Can you work these out from the model? Positions are in its coordinate system, mm. Face numbers are marked on the shaded views. A direction names the side the tool comes from. Coordinates: 2 decimals unless noted, no trailing zeros. Loops run counter-clockwise (first coordinate to the right, second up) from the corner with the lowest first, then second, coordinate; pieces in that order, holes last. Notation, with made-up numbers: (-30, 0.25) -> (-8, 0.25) arc R26 ccw to (-8, 31.25) -> close; hole circle Ø10 at (-36, 30.25). An arc over 180 degrees is marked (long way). Use one line per item in the form item = value. Start each with the question number.
(1) Imagine slicing it at B-B (y = -31). State how many separate pieces and enclosed holes the cut face has, plus the area to 3 significant figures.
(2) Imagine slicing it at A-A (x = 25.5). List the corners of the cut face in (y, z) for me.
(3) Thinking about a two-plate mould opening in X: for the marked faces 1, 2, 3 and 4, which applies, released by +X, released by -X, zero draft, split by the parting line, or undercut?
(4) On a 3-axis mill with a long thin cutter (end or side, diameter ignored), from which of +Z, -Z, +X, -X, +Y, -Y can I reach the whole of each face in a straight line? I mean the marked faces 5, 6, 7 and 8. Say none if no direction works.
(5) I need wall thicknesses on line 1 (X direction, y = -432, z = -107.5); line 2 (Z direction, x = -67, y = -258); line 3 (Z direction, x = -51, y = -216). Which ranges of each line are inside material? Lowest first, please. Write a range as [from, to].
(6) Imagine slicing it at C-C (x = -137). List the corners of the cut face in (y, z) for me.
(7) I'm going to push flat-ended pins straight in: pin 1 (3 mm diameter, centred on x = 83, y = -279, fed in from +Z); pin 2 (1 mm diameter, centred on y = -220.5, z = -128.5, fed in from +X); pin 3 (2 mm diameter, centred on y = -380.5, z = 40.5, fed in from +X). Where does each tip first touch, or does it pass through?
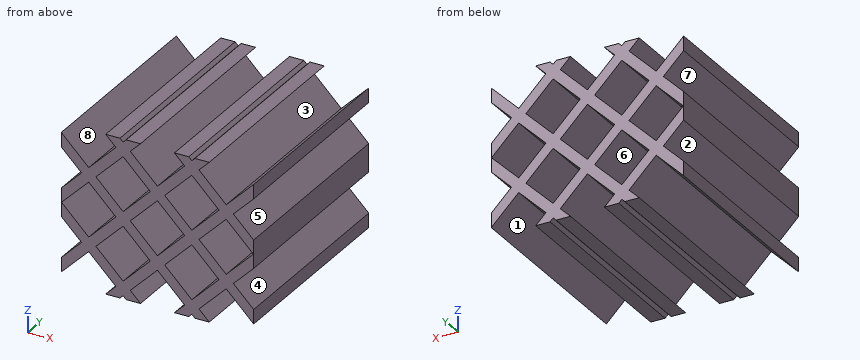
```python
from build123d import *

# Parameters (mm, degrees)
F1_DEPTH = 500


with BuildPart() as f1:
    # F0 (on Front) → F1 (new body)
    with BuildSketch(Plane.XZ):
        Polygon((237.5, 0.619228), (237.5, 34.736111), (187.383297, 84.852814), (237.5, 134.969517), (237.5, 170.324856), (169.705627, 102.530483), (102.530483, 169.705627), (127.824856, 195), (92.469517, 195), (84.852814, 187.383297), (77.236111, 195), (41.880772, 195), (67.175144, 169.705627), (0, 102.530483), (-67.175144, 169.705627), (-41.880772, 195), (-77.236111, 195), (-84.852814, 187.383297), (-92.469517, 195), (-127.824856, 195), (-102.530483, 169.705627), (-169.705627, 102.530483), (-237.5, 170.324856), (-237.5, 134.969517), (-187.383297, 84.852814), (-237.5, 34.736111), (-237.5, 0.619228), (-236.880772, 0), (-237.5, -0.619228), (-237.5, -34.736111), (-187.383297, -84.852814), (-237.5, -134.969517), (-237.5, -170.324856), (-169.705627, -102.530483), (-102.530483, -169.705627), (-127.824856, -195), (-92.469517, -195), (-84.852814, -187.383297), (-77.236111, -195), (-41.880772, -195), (-67.175144, -169.705627), (0, -102.530483), (67.175144, -169.705627), (41.880772, -195), (77.236111, -195), (84.852814, -187.383297), (92.469517, -195), (127.824856, -195), (102.530483, -169.705627), (169.705627, -102.530483), (237.5, -170.324856), (237.5, -134.969517), (187.383297, -84.852814), (237.5, -34.736111), (237.5, -0.619228), (236.880772, 0), align=None)
        Polygon((-17.67767, -84.852814), (-84.852814, -152.027958), (-152.027958, -84.852814), (-84.852814, -17.67767), align=None, mode=Mode.SUBTRACT)
        Polygon((152.027958, -84.852814), (84.852814, -152.027958), (17.67767, -84.852814), (84.852814, -17.67767), align=None, mode=Mode.SUBTRACT)
        Polygon((-169.705627, -67.175144), (-236.880772, 0), (-169.705627, 67.175144), (-102.530483, 0), align=None, mode=Mode.SUBTRACT)
        Polygon((67.175144, 0), (0, -67.175144), (-67.175144, 0), (0, 67.175144), align=None, mode=Mode.SUBTRACT)
        Polygon((-17.67767, 84.852814), (-84.852814, 17.67767), (-152.027958, 84.852814), (-84.852814, 152.027958), align=None, mode=Mode.SUBTRACT)
        Polygon((152.027958, 84.852814), (84.852814, 17.67767), (17.67767, 84.852814), (84.852814, 152.027958), align=None, mode=Mode.SUBTRACT)
        Polygon((169.705627, 67.175144), (236.880772, 0), (169.705627, -67.175144), (102.530483, 0), align=None, mode=Mode.SUBTRACT)
        Polygon((237.5, -0.619228), (237.5, 0.619228), (236.880772, 0), align=None)
        Polygon((-236.880772, 0), (-237.5, 0.619228), (-237.5, -0.619228), align=None)
    extrude(amount=F1_DEPTH)


solid = f1.part
```
Worked out:
q1.separate_pieces = 1
q1.enclosed_holes = 7
q1.area = 66,800 mm2
q2.outline = (-500, -128.03) -> (0, -128.03) -> (0, -92.68) -> (-500, -92.68) -> close; (-500, -77.03) -> (0, -77.03) -> (0, -41.68) -> (-500, -41.68) -> close; (-500, 41.68) -> (0, 41.68) -> (0, 77.03) -> (-500, 77.03) -> close; (-500, 92.68) -> (0, 92.68) -> (0, 128.03) -> (-500, 128.03) -> close
q3.face_1 = undercut
q3.face_2 = released by -X
q3.face_3 = undercut
q3.face_4 = released by +X
q4.face_5 = +X, +Y, -Y
q4.face_6 = +Y, -Y
q4.face_7 = -X, +Y, -Y
q4.face_8 = +Z, +Y, -Y
q5.line_1 = [-210.03, -174.68], [-164.74, -129.38], [-40.32, -4.97], [4.97, 40.32], [129.38, 164.74], [174.68, 210.03]
q5.line_2 = [-195, -169.88], [-169.53, -134.18], [-35.53, -0.18], [0.18, 35.53], [134.18, 169.53], [169.88, 195]
q5.line_3 = [-195, -185.88], [-153.53, -118.18], [-51.53, -16.18], [16.18, 51.53], [118.18, 153.53], [185.88, 195]
q6.outline = (-500, -135.24) -> (0, -135.24) -> (0, -99.88) -> (-500, -99.88) -> close; (-500, -69.82) -> (0, -69.82) -> (0, -34.47) -> (-500, -34.47) -> close; (-500, 34.47) -> (0, 34.47) -> (0, 69.82) -> (-500, 69.82) -> close; (-500, 99.88) -> (0, 99.88) -> (0, 135.24) -> (-500, 135.24) -> close
q7.pin_1 = 190.74
q7.pin_2 = 231.53
q7.pin_3 = 232.74
